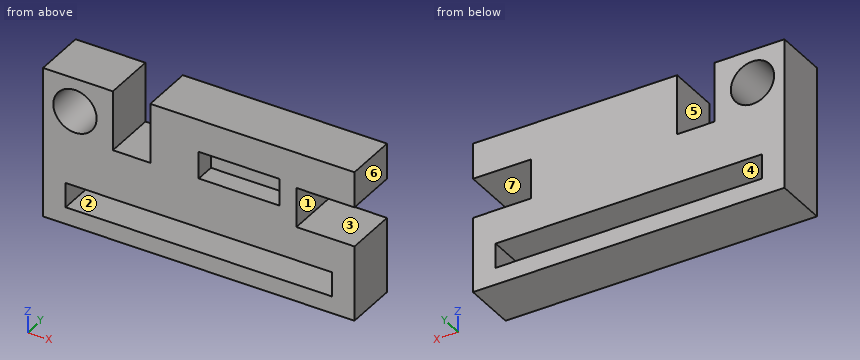
```python
from build123d import *

# Parameters (mm, degrees)
F0_W      = 118.1190237403
F0_H      = 57.0687428117
F1_DEPTH  = 20
F2_R      = 8.2109048963
F3_DEPTH  = 20.001
F4_W      = 14.182465151
F4_H      = 22.6561129093
F5_DEPTH  = 20.001
F6_W      = 30.6975711137
F6_H      = 10.263627395
F7_DEPTH  = 7.5
F8_W      = 22.0171548426
F8_H      = 15.0222154334
F9_DEPTH  = 20.001
F10_W     = 100.9567603469
F10_H     = 9.3305669725
F11_DEPTH = 20.001


with BuildPart() as f1:
    # F0 (on Front) → F1 (new body)
    with BuildSketch(Plane.XZ):
        Rectangle(F0_W, F0_H)
    extrude(amount=F1_DEPTH)

    # F2 (on face) → F3 (cut, through all)
    with BuildSketch(Plane.XZ.offset(20)):
        with Locations((-46.9327643514, 15.955273062)):
            Circle(F2_R)
    extrude(amount=-F3_DEPTH, mode=Mode.SUBTRACT)

    # F4 (on face) → F5 (cut, through all)
    with BuildSketch(Plane.XZ.offset(20)):
        with Locations((-25.4724537954, 17.2063149512)):
            Rectangle(F4_W, F4_H)
    extrude(amount=-F5_DEPTH, mode=Mode.SUBTRACT)

    # F6 (on face) → F7 (cut)
    with BuildSketch(Plane.XZ.offset(20)):
        with Locations((15.3487855569, 11.196683161)):
            Rectangle(F6_W, F6_H)
    extrude(amount=-F7_DEPTH, mode=Mode.SUBTRACT)

    # F8 (on face) → F9 (cut, through all)
    with BuildSketch(Plane.XZ.offset(20)):
        with Locations((48.0509344488, 7.5111077167)):
            Rectangle(F8_W, F8_H)
    extrude(amount=-F9_DEPTH, mode=Mode.SUBTRACT)

    # F10 (on face) → F11 (cut, through all)
    with BuildSketch(Plane.XZ.offset(20)):
        with Locations((0, -17.4481645226)):
            Rectangle(F10_W, F10_H)
    extrude(amount=-F11_DEPTH, mode=Mode.SUBTRACT)


solid = f1.part
```
Could you check a few things on this model? Use its own coordinates, in mm. Face numbers are marked on the shaded views. A direction names the side the tool comes from. Give positions to 0.01 mm unless a question says otherwise; leave off trailing zeros. Order: outer loops, then holes, each group sorted by start corner. A loop starts at its lowest first (then second) coordinate and runs counter-clockwise, first axis right, second up.
Q1. Suppose I cut it at D-D, the plane z = 12. Write out the boundary of the cut face in (x, y), and give its area (3 significant figures).
Q2. For the marked faces 5, 6 and 7, which set-ups out of +Z, -Z, +X, -X, +Y, -Y let a thin tool reach every point of the face, with its end or its side?
Q3. Suppose I cut it at A-A, the plane z = 25.5. Write out the boundary of the cut face in (x, y), and give its area (3 significant figures).
Q4. Suppose I cut it at C-C, the plane x = 49. Write out the boundary of the cut face in (y, z), and give its area (3 significant figures).
Q5. Suppose I cut it at B-B, the plane x = -20. Write out the boundary of the cut face in (y, z).
Q6. If I drill on line 1 along X through (y, z) = (-13.5, 15.5); line 2 along X through (y, z) = (-17.5, 7.5); line 3 along Z through (x, y) = (8, -15.5), over which ranges is the centre line in solid material (lowest first)?
Q7. I'm going to push flat-ended pins straight in: P1, Ø8, axis at x = 12.5, z = 10.5, coming from the -Y side; P2, Ø10, axis at x = -26, y = -7, coming from the +Z side; P3, Ø1, axis at y = -17.5, z = 8, coming from the +X side. Where does each tip first touch, or does it pass through?
Q8. We'd pull the mould along X, two halves only. Please class the marked faces 1, 2, 3 and 4: +X half, -X half, draft (parallel to the pull), parting line (faces both ways), or undercut.
Solution:
1. outline: (-59.06, -20) - (-54.13, -20) - (-54.13, 0) - (-59.06, 0) - close; (-39.74, -20) - (-32.56, -20) - (-32.56, 0) - (-39.74, 0) - close; (-18.38, -20) - (0, -20) - (0, -12.5) - (30.7, -12.5) - (30.7, -20) - (37.04, -20) - (37.04, 0) - (-18.38, 0) - close
1. area: 1,120 mm2
2. face 5: +Z, +Y, -Y
2. face 6: +Z, -Z, +X, +Y, -Y
2. face 7: +X, +Y, -Y
3. outline: (-59.06, -20) - (-32.56, -20) - (-32.56, 0) - (-59.06, 0) - close; (-18.38, -20) - (59.06, -20) - (59.06, 0) - (-18.38, 0) - close
3. area: 2,080 mm2
4. outline: (-20, -28.53) - (0, -28.53) - (0, -22.11) - (-20, -22.11) - close; (-20, -12.78) - (0, -12.78) - (0, 0) - (-20, 0) - close; (-20, 15.02) - (0, 15.02) - (0, 28.53) - (-20, 28.53) - close
4. area: 654 mm2
5. outline: (-20, -28.53) - (0, -28.53) - (0, -22.11) - (-20, -22.11) - close; (-20, -12.78) - (0, -12.78) - (0, 5.88) - (-20, 5.88) - close
6. line 1: x = -59.06 to -55.13, -38.73 to -32.56, -18.38 to 0, 30.7 to 59.06
6. line 2: x = -59.06 to -32.56, -18.38 to 0, 30.7 to 37.04
6. line 3: z = -28.53 to -22.11, -12.78 to 6.06, 16.33 to 28.53
7. P1: stops at y = -12.5
7. P2: stops at z = 5.88
7. P3: stops at x = 37.04
8. face 1: +X half
8. face 2: undercut
8. face 3: draft
8. face 4: undercut
